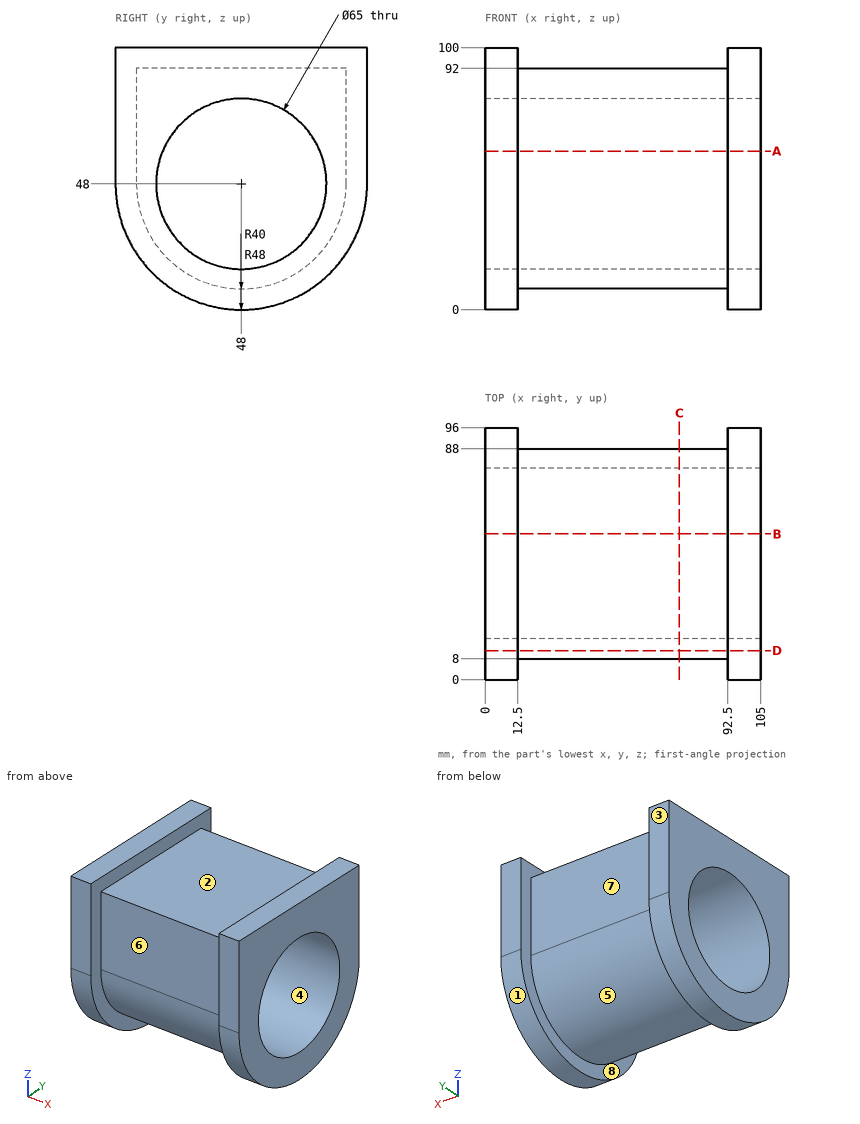
Source: three-view drawing plus pictorial views. Frame: mm from the lowest corner of the part. A direction names the side the tool comes from. Round coordinates to 2 decimals unless told otherwise and drop trailing zeros. Loops run counter-clockwise (first coordinate to the right, second up) from the corner with the lowest first, then second, coordinate; pieces in that order, holes last. Notation, with made-up numbers: M 69.25,31.25 L 107.25,31.25 A13 ccw 107.25,53.25 Z; hole C -30,1 d1. An arc over 180 degrees is marked long. Put each result on its own line as item: value.
(1) Section C-C, the plane x = 74. Return loops of the section in (y, z).
Solutions:
outline: M 8,48 A40 ccw 88,48 L 88,92 L 8,92 Z; hole C 48,48 d65
(2) Section D-D, the plane y = 11. Return loops of the section in (x, z).
Solutions:
outline: M 0,17.42 L 12.5,17.42 L 12.5,32.8 L 92.5,32.8 L 92.5,17.42 L 105,17.42 L 105,100 L 92.5,100 L 92.5,92 L 12.5,92 L 12.5,100 L 0,100 Z
(3) First-contact query: pin 1 (4 mm diameter, centred on x = 77.5, z = 43.5, fed in from +Y); pin 2 (3 mm diameter, centred on x = 88, z = 55.5, fed in from +Y); pin 3 (5 mm diameter, centred on x = 43.5, z = 53.5, fed in from -Y). Flat tips, straight axial feed; report the tip coordinate or a pass-through.
Solutions:
pin 1: y = 87.92
pin 2: y = 88
pin 3: y = 8
(4) Access query for the marked faces 5, 6, 7 and 8. Directions: +Z, -Z, +X, -X, +Y, -Y. A direction counts if a zero-diameter tool reaches every point of the face in a straight line with its end or side. Return the directions, or none.
Solutions:
face 5: -Z
face 6: +Z, -Z, -Y
face 7: +Z, -Z, +Y
face 8: none
(5) Ray query, line 1 (Y direction, x = 54, z = 48); line 2 (X direction, y = 74, z = 17); line 3 (Z direction, x = 51.5, y = 43). Return the intervals inside material, ascending. Write a range as [from, to].
Solutions:
line 1: [8, 15.5], [80.5, 88]
line 2: [0, 12.5], [92.5, 105]
line 3: [8.31, 15.89], [80.11, 92]
(6) Pull-direction query (Z, two-part tool) for the marked faces 1, 2, 3 and 4; classes: released by +Z, released by -Z, zero draft, split by the parting line, or undercut.
Solutions:
face 1: released by -Z
face 2: released by +Z
face 3: zero draft
face 4: undercut
(7) Section A-A, the plane z = 60.5. Return loops of the section in (x, y).
Solutions:
outline: M 0,0 L 12.5,0 L 12.5,8 L 92.5,8 L 92.5,0 L 105,0 L 105,18 L 0,18 Z; M 0,78 L 105,78 L 105,96 L 92.5,96 L 92.5,88 L 12.5,88 L 12.5,96 L 0,96 Z
(8) Section B-B, the plane y = 55.5. Return loops of the section in (x, z).
Solutions:
outline: M 0,0.59 L 12.5,0.59 L 12.5,8.71 L 92.5,8.71 L 92.5,0.59 L 105,0.59 L 105,16.38 L 0,16.38 Z; M 0,79.62 L 105,79.62 L 105,100 L 92.5,100 L 92.5,92 L 12.5,92 L 12.5,100 L 0,100 Z
